```python
from build123d import *

# Parameters (mm, degrees)
F0_R     = 104.775
F1_DEPTH = 6.35
F2_D     = 29.718
F3_D     = 29.718
F4_D     = 29.718
F5_D     = 29.718
F6_D     = 16.6116
F7_D     = 16.6116
F8_D     = 16.6116
F9_D     = 16.6116


with BuildPart() as f1:
    # F0 (on Top) → F1 (new body)
    with BuildSketch(Plane.XY):
        Circle(F0_R)
    extrude(amount=F1_DEPTH)

    # F2 (through all)
    with Locations(Plane(origin=(0, 0, 0), x_dir=(1, 0, 0), z_dir=(0, 0, -1))):
        with Locations((-26.940768, 26.940768)):
            Hole(F2_D / 2)

    # F3 (through all)
    with Locations(Plane(origin=(0, 0, 0), x_dir=(1, 0, 0), z_dir=(0, 0, -1))):
        with Locations((26.940768, 26.940768)):
            Hole(F3_D / 2)

    # F4 (through all)
    with Locations(Plane(origin=(0, 0, 0), x_dir=(1, 0, 0), z_dir=(0, 0, -1))):
        with Locations((-26.940768, -26.940768)):
            Hole(F4_D / 2)

    # F5 (through all)
    with Locations(Plane(origin=(0, 0, 0), x_dir=(1, 0, 0), z_dir=(0, 0, -1))):
        with Locations((26.940768, -26.940768)):
            Hole(F5_D / 2)

    # F6 (through all)
    with Locations(Plane(origin=(0, 0, 0), x_dir=(1, 0, 0), z_dir=(0, 0, -1))):
        with Locations((-53.881537, 53.881537)):
            Hole(F6_D / 2)

    # F7 (through all)
    with Locations(Plane(origin=(0, 0, 0), x_dir=(1, 0, 0), z_dir=(0, 0, -1))):
        with Locations((53.881537, 53.881537)):
            Hole(F7_D / 2)

    # F8 (through all)
    with Locations(Plane(origin=(0, 0, 0), x_dir=(1, 0, 0), z_dir=(0, 0, -1))):
        with Locations((-53.881537, -53.881537)):
            Hole(F8_D / 2)

    # F9 (through all)
    with Locations(Plane(origin=(0, 0, 0), x_dir=(1, 0, 0), z_dir=(0, 0, -1))):
        with Locations((53.881537, -53.881537)):
            Hole(F9_D / 2)


solid = f1.part
```
Design review of the part built by this model. Coordinates are the model's own, in mm. Coordinates: 2 decimals unless noted, no trailing zeros. Loops run counter-clockwise (first coordinate to the right, second up) from the corner with the lowest first, then second, coordinate; pieces in that order, holes last. Notation, with made-up numbers: (31, -19.75) - (55, -19.75) arc R20 ccw to (55, -8.75) - close; hole circle Ø6 at (59, 30.25). An arc over 180 degrees is marked (long way). Use CSV: the item, a comma, the result in double quotes. Start each with the question number.
1) Consider section C-C on z = 2. Give the number of separate pieces and of enclosed holes in the cut face, then the cut area to 3 significant figures.
2) The part is to be moulded in two halves that separate along X. For faces 1 (the flat face through (-1, 1, 0)), 2 (the cylindrical face through (-34.93, -39.47, 3.22)), 3 (the cylindrical face through (-22.713, -102.283, 3.131)), say which applies: +X half, -X half, draft (parallel to the pull), parting line (faces both ways), or undercut.
3) Consider section D-D on x = -71.5. Write out the cut boundary in (y, z), then the cut area to 3 significant figures.
4) Consider section A-A on x = -27.5. Write out the cut boundary in (y, z).
5) For pin 1 Ø13.5 at (x, y) = (-53.88, -53.88) entering from -Z; pin 2 Ø1 at (y, z) = (81, 5) entering from -X, all flat-tipped, find the tip position at first contact; note any pin that passes through.
6) Consider section B-B on y = 50.5. Write out the cut boundary in (x, z), then the cut area to 3 significant figures.
7) Wall thickness on L1, parallel to X at y = -19, z = 3; L2, parallel to X at y = 35.5, z = 3; L3, parallel to Y at x = -47, z = 6: over which ranges is each line inside the solid? List them lowest first. Write a range as from..to.
Geometry says:
1,separate pieces,"1"
1,enclosed holes,"8"
1,area,"30,800 mm^2"
2,face 1,"draft"
2,face 2,"undercut"
2,face 3,"parting line"
3,outline,"(-76.59, 0) - (76.59, 0) - (76.59, 6.35) - (-76.59, 6.35) - close"
3,area,"973 mm^2"
4,outline,"(-101.1, 0) - (-41.79, 0) - (-41.79, 6.35) - (-101.1, 6.35) - close; (-12.09, 0) - (12.09, 0) - (12.09, 6.35) - (-12.09, 6.35) - close; (41.79, 0) - (101.1, 0) - (101.1, 6.35) - (41.79, 6.35) - close"
5,pin 1,"through"
5,pin 2,"x = -67.06"
6,outline,"(-91.8, 0) - (-61.47, 0) - (-61.47, 6.35) - (-91.8, 6.35) - close; (-46.3, 0) - (46.3, 0) - (46.3, 6.35) - (-46.3, 6.35) - close; (61.47, 0) - (91.8, 0) - (91.8, 6.35) - (61.47, 6.35) - close"
6,area,"973 mm^2"
7,L1,"-103.04..-39.5, -14.38..14.38, 39.5..103.04"
7,L2,"-98.58..-39.09, -14.79..14.79, 39.09..98.58"
7,L3,"-93.64..-58.53, -49.23..49.23, 58.53..93.64"
